CAD build for the part. Positions are in the model's coordinates, mm. A direction names the side the tool comes from. Round coordinates to 2 decimals unless told otherwise and drop trailing zeros. Loops run counter-clockwise (first coordinate to the right, second up) from the corner with the lowest first, then second, coordinate; pieces in that order, holes last.
from build123d import *

# Parameters (mm, degrees)
F0_R     = 82.55
F1_DEPTH = 50.8
F2_R     = 3.81
F3_W     = 38.1
F3_H     = 12.7
F4_DEPTH = 50.8


with BuildPart() as f1:
    # F0 (on Right) → F1 (new body)
    with BuildSketch(Plane.YZ):
        Circle(F0_R)
    extrude(amount=F1_DEPTH)

    # F2
    f2_edges = [f1.edges().sort_by_distance(p)[0] for p in [
        (50.8, -82.55, 0),
        (0, -82.55, 0),
    ]]
    fillet(f2_edges, radius=F2_R)

    # F3 (on face) → F4 (join)
    with BuildSketch(Plane(origin=(0, 0, 0), x_dir=(0, -1, 0), z_dir=(-1, 0, 0))):
        Rectangle(F3_W, F3_H)
    extrude(amount=F4_DEPTH)


solid = f1.part
Item 1: Cut at D-D (x = -39). List the corners of the cut face in (y, z).
Verdict:
outline: (-19.05, -6.35) - (19.05, -6.35) - (19.05, 6.35) - (-19.05, 6.35) - close
Item 2: Cut at A-A (y = 0). List the corners of the cut face in (x, z), plus the area to 3 significant figures.
Verdict:
outline: (-50.8, -6.35) - (0, -6.35) - (0, -78.74) arc R3.81 ccw to (3.81, -82.55) - (46.99, -82.55) arc R3.81 ccw to (50.8, -78.74) - (50.8, 78.74) arc R3.81 ccw to (46.99, 82.55) - (3.81, 82.55) arc R3.81 ccw to (0, 78.74) - (0, 6.35) - (-50.8, 6.35) - close
area: 9,020 mm2
Item 3: 3-axis set-ups, long thin cutter, end or side, ignore diameter. For faces 1 (the flat face through (-25, 0, -6.35)), 2 (the flat face through (-25, -19.05, 0)), 3 (the flat face through (-25, 0, 6.35)), 4 (the flat face through (-25, 19.05, 0)): which of +Z, -Z, +X, -X, +Y, -Y reach the whole face in a straight line?
Verdict:
face 1: -Z, -X, +Y, -Y
face 2: +Z, -Z, -X, -Y
face 3: +Z, -X, +Y, -Y
face 4: +Z, -Z, -X, +Y
Item 4: Flat gauge pins, fed straight in: P1, Ø12, axis at x = 38, y = -24.5, coming from the +Z side; P2, Ø2, axis at x = 24.5, y = 51.5, coming from the +Z side; P3, Ø2, axis at y = -36.5, z = -20, coming from the -X side. Where does each tip first touch, or does it go through?
Verdict:
P1: stops at z = 80.45
P2: stops at z = 65.3
P3: stops at x = 0
Item 5: Cut at B-B (z = 0). List the corners of the cut face in (x, y).
Verdict:
outline: (-50.8, -19.05) - (0, -19.05) - (0, -78.74) arc R3.81 ccw to (3.81, -82.55) - (46.99, -82.55) arc R3.81 ccw to (50.8, -78.74) - (50.8, 78.74) arc R3.81 ccw to (46.99, 82.55) - (3.81, 82.55) arc R3.81 ccw to (0, 78.74) - (0, 19.05) - (-50.8, 19.05) - close
Item 6: Cut at C-C (x = 20.5). List the corners of the cut face in (y, z), plus the area to 3 significant figures.
Verdict:
outline: circle Ø165.1 at (0, 0)
area: 21,400 mm2
Item 7: Wall check: L1, parallel to X at y = 31, z = -10; L2, parallel to Z at x = -7, y = -10.5; L3, parallel to Z at x = 36, y = 0.5. Give the ranges that are in metal, low to high.
Verdict:
L1: x = 0 to 50.8
L2: z = -6.35 to 6.35
L3: z = -82.55 to 82.55
